Geometry: final body of the model. Coordinates: model frame, mm. Face numbers are marked on the shaded views. A direction names the side the tool comes from. Give positions to 0.01 mm unless a question says otherwise; leave off trailing zeros. Write each loop counter-clockwise with the first axis right and the second up, starting at its lowest first coordinate (ties: lowest second). Pieces come first, ordered by that corner, then holes.
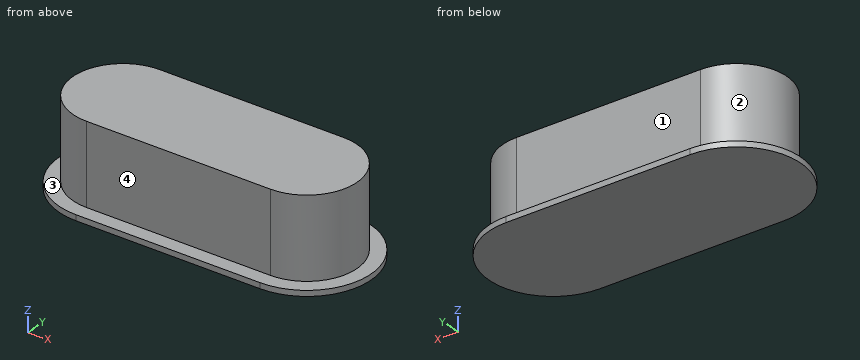
```python
from build123d import *

# Parameters (mm, degrees)
F1_DEPTH = 2.85
F3_DEPTH = 0.2


with BuildPart() as f1:
    # F0 (on Top) → F1 (new body)
    with BuildSketch(Plane.XY):
        with BuildLine():
            Line((-3.225, -1.775), (3.225, -1.775))
            ThreePointArc((3.225, -1.775), (5, 0), (3.225, 1.775))
            Line((3.225, 1.775), (-3.225, 1.775))
            ThreePointArc((-3.225, 1.775), (-5, 0), (-3.225, -1.775))
        make_face()
    extrude(amount=F1_DEPTH)

    # F2 (on face) → F3 (join)
    with BuildSketch(Plane(origin=(0, 0, 0), x_dir=(1, 0, 0), z_dir=(0, 0, -1))):
        with BuildLine():
            Line((-3.225, -2.275), (3.225, -2.275))
            ThreePointArc((3.225, -2.275), (5.5, 0), (3.225, 2.275))
            Line((3.225, 2.275), (-3.225, 2.275))
            ThreePointArc((-3.225, 2.275), (-5.5, 0), (-3.225, -2.275))
        make_face()
    extrude(amount=F3_DEPTH)


solid = f1.part
```
Item 1: Section A-A, the plane x = -1.25. Return the cut outline in (y, z) (3 decimals).
Found:
outline: (-2.275, -0.2) - (2.275, -0.2) - (2.275, 0) - (1.775, 0) - (1.775, 2.85) - (-1.775, 2.85) - (-1.775, 0) - (-2.275, 0) - close
Item 2: Section C-C, the plane z = 2.2. Return the cut outline in (x, y) (3 decimals).
Found:
outline: (-3.225, -1.775) - (3.225, -1.775) arc R1.775 ccw to (3.225, 1.775) - (-3.225, 1.775) arc R1.775 ccw to start
Item 3: Line query: L1, parallel to Y at x = -2.25, z = 1.15 (3 decimals); L2, parallel to X at y = -1.35, z = 1.5; L3, parallel to X at y = -0.1, z = 0.65. Output: solid intervals per line, ascending.
Found:
L1: y = -1.775 to 1.775
L2: x = -4.38 to 4.38
L3: x = -5 to 5
Item 4: Pin query (flat end, axial travel): pin 1 Ø1.5 at (y, z) = (-1, 1.5) entering from +X; pin 2 Ø1.4 at (x, z) = (0.5, 1.5) entering from +Y (3 decimals); pin 3 Ø1 at (y, z) = (-1.5, 2) entering from +X. Return the tip coordinate at first contact, or that it passes through.
Found:
pin 1: stops at x = 4.98
pin 2: stops at y = 1.775
pin 3: stops at x = 4.69
Item 5: Reachability of the marked faces 1, 2, 3 and 4 from +Z, -Z, +X, -X, +Y, -Y: full face, straight path, thin tool, end or side. Return the list, or none.
Found:
face 1: +Z, +X, -X, +Y
face 2: +Z, -X
face 3: +Z
face 4: +Z, +X, -X, -Y
Item 6: Section B-B, the plane y = 0. Return the cut outline in (x, z), plus the area to 3 significant figures.
Found:
outline: (-5.5, -0.2) - (5.5, -0.2) - (5.5, 0) - (5, 0) - (5, 2.85) - (-5, 2.85) - (-5, 0) - (-5.5, 0) - close
area: 30.7 mm2
